Could you check a few things on this model? Use its own coordinates, in mm. Coordinates: 2 decimals unless noted, no trailing zeros. Loops run counter-clockwise (first coordinate to the right, second up) from the corner with the lowest first, then second, coordinate; pieces in that order, holes last.
1) If I drill on line 1 along X through (y, z) = (7, 2.75); line 2 along X through (y, z) = (13.5, 3.25); line 3 along Y through (x, z) = (8.5, 6), over which ranges is the centre line in solid material (lowest first)?
2) Thinking about a two-plate mould opening in Y: for faces 1 (the face through (-0.47, -44.76, 3.94)), 2 (the face through (13.694, -8.123, 3.944)), 3 (the face through (9, -7, 8)), 4 (the face through (39, 21.97, 3.94)), which applies, released by +Y, released by -Y, zero draft, split by the parting line, or undercut?
3) Imagine slicing it at D-D on z = 2. Please give me the cut outline in (x, y), plus the area to 3 significant figures.
4) Imagine slicing it at C-C on y = 13. Please give me the cut outline in (x, z), plus the area to 3 significant figures.
5) Imagine slicing it at B-B on y = -24.5. Please give me the cut outline in (x, z), plus the area to 3 significant figures.
6) Imagine slicing it at A-A on x = -21. Please give me the cut outline in (y, z), plus the area to 3 significant figures.
7) Will these pins go through, and if not, where does the flat tip stop? P1, Ø2, axis at x = 21.5, z = 5.5, coming from the +Y side; P2, Ø4, axis at x = 11.5, z = 2.5, coming from the +Y side.
```python
from build123d import *

# Parameters (mm, degrees)
F1_DEPTH = 8


with BuildPart() as f1:
    # F0 (on Top) → F1 (new body)
    with BuildSketch(Plane.XY):
        with BuildLine():
            ThreePointArc((11, -28.76845), (7.778175, -20.990275), (0, -17.76845))
            ThreePointArc((0, -17.76845), (-7.778175, -36.546625), (11, -28.76845))
        make_face()
        with BuildLine():
            ThreePointArc((-13.914208, 14.384225), (-35.539393, 17.231234), (-15.387929, 8.884225))
            ThreePointArc((-15.387929, 8.884225), (-14.289024, 11.537215), (-13.914208, 14.384225))
        make_face()
        with BuildLine():
            ThreePointArc((35.914208, 14.384225), (22.067199, 25.009409), (15.387929, 8.884225))
            ThreePointArc((15.387929, 8.884225), (27.761218, 3.759041), (35.914208, 14.384225))
        make_face()
        with BuildLine():
            ThreePointArc((24.914208, -1.615775), (38.770615, 22.384225), (11.057802, 22.384225))
            ThreePointArc((11.057802, 22.384225), (0, 16), (-11.057802, 22.384225))
            ThreePointArc((-11.057802, 22.384225), (-38.770615, 22.384225), (-24.914208, -1.615775))
            ThreePointArc((-24.914208, -1.615775), (-13.856406, -8), (-13.856406, -20.76845))
            ThreePointArc((-13.856406, -20.76845), (0, -44.76845), (13.856406, -20.76845))
            ThreePointArc((13.856406, -20.76845), (13.786503, -7.959641), (24.914208, -1.615775))
        make_face()
        with BuildLine():
            ThreePointArc((11, -28.76845), (-7.778175, -36.546625), (0, -17.76845))
            ThreePointArc((0, -17.76845), (7.778175, -20.990275), (11, -28.76845))
        make_face(mode=Mode.SUBTRACT)
        with BuildLine():
            ThreePointArc((-13.914208, 14.384225), (-14.289024, 11.537215), (-15.387929, 8.884225))
            ThreePointArc((-15.387929, 8.884225), (-35.539393, 17.231234), (-13.914208, 14.384225))
        make_face(mode=Mode.SUBTRACT)
        with BuildLine():
            ThreePointArc((11, 0), (7.778175, -7.778175), (0, -11))
            ThreePointArc((0, -11), (-9.526279, -5.5), (-9.526279, 5.5))
            ThreePointArc((-9.526279, 5.5), (0, 11), (9.526279, 5.5))
            ThreePointArc((9.526279, 5.5), (10.625184, 2.847009), (11, 0))
        make_face(mode=Mode.SUBTRACT)
        with BuildLine():
            ThreePointArc((35.914208, 14.384225), (27.761218, 3.759041), (15.387929, 8.884225))
            ThreePointArc((15.387929, 8.884225), (22.067199, 25.009409), (35.914208, 14.384225))
        make_face(mode=Mode.SUBTRACT)
    extrude(amount=F1_DEPTH)


solid = f1.part
```
Filled in:
1. line 1: x = -39.11 to -33.07, -16.76 to -8.49, 8.49 to 16.76, 33.07 to 39.11
1. line 2: x = -40.89 to -35.88, -13.95 to 13.95, 35.88 to 40.89
1. line 3: y = -42.32 to -35.75, -21.79 to -6.98, 6.98 to 19.24
2. face 1: undercut
2. face 2: undercut
2. face 3: zero draft
2. face 4: split by the parting line
3. outline: (-24.91, -1.62) arc R12.77 cw to (-13.86, -20.77) arc R16 ccw (long way) to (13.86, -20.77) arc R12.69 cw to (24.91, -1.62) arc R16 ccw (long way) to (11.06, 22.38) arc R12.77 cw to (-11.06, 22.38) arc R16 ccw (long way) to start; hole (-15.39, 8.88) arc R11 ccw to (-13.91, 14.38) arc R11 ccw (long way) to start; hole (0, -17.77) arc R11 ccw (long way) to (11, -28.77) arc R11 ccw to start; hole (0, -11) arc R11 ccw to (11, 0) arc R11 ccw (long way) to start; hole circle Ø22 at (24.91, 14.38)
3. area: 1,720 mm2
4. outline: (-40.85, 0) - (-35.83, 0) - (-35.83, 8) - (-40.85, 8) - close; (-14, 0) - (14, 0) - (14, 8) - (-14, 8) - close; (35.83, 0) - (40.85, 0) - (40.85, 8) - (35.83, 8) - close
4. area: 304 mm2
5. outline: (-15.42, 0) - (-10.14, 0) - (-10.14, 8) - (-15.42, 8) - close; (10.14, 0) - (15.42, 0) - (15.42, 8) - (10.14, 8) - close
5. area: 84.5 mm2
6. outline: (-2.23, 0) - (4.1, 0) - (4.1, 8) - (-2.23, 8) - close; (24.66, 0) - (29.9, 0) - (29.9, 8) - (24.66, 8) - close
6. area: 92.5 mm2
7. P1: stops at y = 30.2
7. P2: stops at y = 25.6
